Geometry: final body of the model. Coordinates: model frame, mm. A direction names the side the tool comes from. Give positions to 0.01 mm unless a question says otherwise; leave off trailing zeros. Loops run counter-clockwise (first coordinate to the right, second up) from the corner with the lowest first, then second, coordinate; pieces in that order, holes last. Notation, with made-up numbers: (54.25, 29) - (72.25, 29) arc R20 ccw to (72.25, 65) - close; hole circle Ø5 at (40, 58). An arc over 180 degrees is marked (long way). Answer in a Markdown table with one row per item.
from build123d import *

# Parameters (mm, degrees)
SKETCH3_W           = 25
SKETCH3_H           = 17
BOSS_EXTRUDE3_DEPTH = 1.3
SKETCH4_W           = 4.047255343
SKETCH4_H           = 0.65
CUT_EXTRUDE1_DEPTH  = 30.3
SKETCH6_W           = 23.5
SKETCH6_H           = 13
BOSS_EXTRUDE4_DEPTH = 0.1
BOSS_EXTRUDE6_DEPTH = 0.05


with BuildPart() as part:
    # Sketch3 → Boss-Extrude3 (new body)
    with BuildSketch(Plane(origin=(0, 0, 0), x_dir=(1, 0, 0), z_dir=(0, 1, 0))):
        with Locations((0, -12.92)):
            Rectangle(SKETCH3_W, SKETCH3_H)
    extrude(amount=BOSS_EXTRUDE3_DEPTH)

    # Sketch4 → Cut-Extrude1 (cut)
    with BuildSketch(Plane.ZY.offset(12.5)):
        with Locations((21.656372328, 1.525)):
            Rectangle(SKETCH4_W, SKETCH4_H)
    extrude(amount=-CUT_EXTRUDE1_DEPTH, mode=Mode.SUBTRACT)

    # Sketch6 → Boss-Extrude4 (add)
    with BuildSketch(Plane(origin=(0, 1.3, 0), x_dir=(1, 0, 0), z_dir=(0, 1, 0))):
        with Locations((0, -11.67)):
            Rectangle(SKETCH6_W, SKETCH6_H)
    extrude(amount=BOSS_EXTRUDE4_DEPTH)

    # Sketch10 → Boss-Extrude6 (add)
    with BuildSketch(Plane(origin=(0, 1.3, 0), x_dir=(1, 0, 0), z_dir=(0, 1, 0))):
        with BuildLine():
            Line((-5, -21.82), (-5, -22.06))
            Line((-5, -22.06), (5, -22.06))
            Line((5, -22.06), (5, -21.82))
            ThreePointArc((5, -21.82), (5.058578644, -21.678578644), (5.2, -21.62))
            Line((5.2, -21.62), (7.3, -21.62))
            ThreePointArc((7.3, -21.62), (7.441421356, -21.561421356), (7.5, -21.42))
            Line((7.5, -21.42), (7.5, -18.82))
            ThreePointArc((7.5, -18.82), (7.441421356, -18.678578644), (7.3, -18.62))
            Line((7.3, -18.62), (-7.3, -18.62))
            ThreePointArc((-7.3, -18.62), (-7.441421356, -18.678578644), (-7.5, -18.82))
            Line((-7.5, -18.82), (-7.5, -21.42))
            ThreePointArc((-7.5, -21.42), (-7.441421356, -21.561421356), (-7.3, -21.62))
            Line((-7.3, -21.62), (-5.2, -21.62))
            ThreePointArc((-5.2, -21.62), (-5.058578644, -21.678578644), (-5, -21.82))
        make_face()
    extrude(amount=BOSS_EXTRUDE6_DEPTH)


solid = part.part
Q1. First-contact query: pin 1 (2 mm diameter, centred on x = 3, z = 21, fed in from +Y). Flat tip, straight axial feed; report the tip coordinate or a pass-through.
Check values:
| item | result |
|---|---|
| pin 1 | y = 1.35 |
Q2. Cut plane B-B (y = 0.8). Output: boundary loops of the cut face in (x, z), and give its area (3 significant figures).
Check values:
| item | result |
|---|---|
| outline | (-12.5, 4.42) - (12.5, 4.42) - (12.5, 21.42) - (-12.5, 21.42) - close |
| area | 425 mm² |
Q3. Material intervals for line 1 along Z through (x, y) = (10.75, 0.6); line 2 along Y through (x, z) = (-9.75, 19.5); line 3 along Y through (x, z) = (-6.5, 19.25), sorted ascending.
Check values:
| item | result |
|---|---|
| line 1 | 4.42 to 21.42 |
| line 2 | 0 to 1.3 |
| line 3 | 0 to 1.35 |
Q4. Cut plane A-A (x = -9). Output: boundary loops of the cut face in (y, z), and give its area (3 significant figures).
Check values:
| item | result |
|---|---|
| outline | (0, 4.42) - (1.3, 4.42) - (1.3, 5.17) - (1.4, 5.17) - (1.4, 18.17) - (1.3, 18.17) - (1.3, 19.63) - (1.2, 19.63) - (1.2, 21.42) - (0, 21.42) - close |
| area | 23.2 mm² |
Q5. Reachability of faces 1 (the flat face through (0, 1.35, 19)), 2 (the flat face through (0, 1, 21.42)), 3 (the flat face through (0, 0, 13)) from +Z, -Z, +X, -X, +Y, -Y: full face, straight path, thin tool, end or side. Return the list, or none.
Check values:
| item | result |
|---|---|
| face 1 | +Z, +X, -X, +Y |
| face 2 | +Z, +X, -X, -Y |
| face 3 | +Z, -Z, +X, -X, -Y |
Q6. Cut plane C-C (x = -4.5). Output: boundary loops of the cut face in (y, z).
Check values:
| item | result |
|---|---|
| outline | (0, 4.42) - (1.3, 4.42) - (1.3, 5.17) - (1.4, 5.17) - (1.4, 18.17) - (1.3, 18.17) - (1.3, 18.62) - (1.35, 18.62) - (1.35, 22.06) - (1.3, 22.06) - (1.3, 19.63) - (1.2, 19.63) - (1.2, 21.42) - (0, 21.42) - close |
